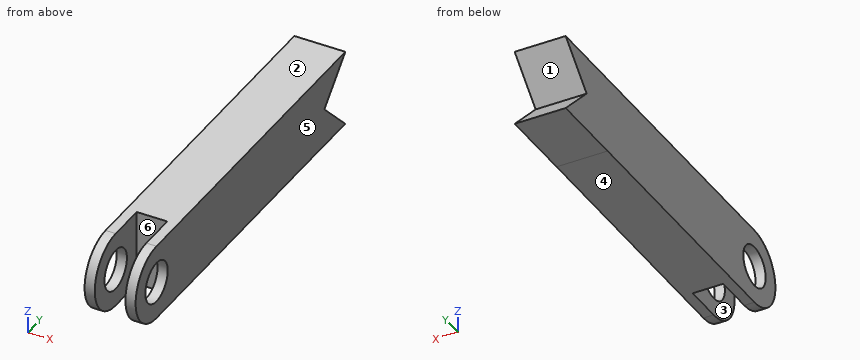
```python
from build123d import *

# Parameters (mm, degrees)
BOSS_EXTRUDE1_DEPTH = 100
CUT_EXTRUDE2_DEPTH  = 20
CUT_EXTRUDE3_START  = -20
CUT_EXTRUDE3_DEPTH  = 20
SKETCH10_R          = 40
BOSS_EXTRUDE6_DEPTH = 20
BOSS_EXTRUDE7_START = 20
SKETCH11_R          = 40
BOSS_EXTRUDE7_DEPTH = 20
SKETCH19_R          = 40
CUT_EXTRUDE7_DEPTH  = 285
SKETCH16_W          = 60
SKETCH16_H          = 150
CUT_EXTRUDE8_DEPTH  = 285
SKETCH20_W          = 100
SKETCH20_H          = 295.959975124
CUT_EXTRUDE9_DEPTH  = 285
BOSS_EXTRUDE8_DEPTH = 100


with BuildPart() as part:
    # Sketch1 → Boss-Extrude1 (new body)
    with BuildSketch(Plane(origin=(0, 0, 0), x_dir=(0, 0, -1), z_dir=(1, 0, 0))):
        with BuildLine():
            Line((-74.767803634, 0), (-74.767803634, 600))
            ThreePointArc((-74.767803634, 600), (0, 674.767803634), (74.767803634, 600))
            Line((74.767803634, 600), (74.767803634, 0))
            ThreePointArc((74.767803634, 0), (0, -74.767803634), (-74.767803634, 0))
        make_face()
    extrude(amount=BOSS_EXTRUDE1_DEPTH)

    # Sketch8 → Cut-Extrude2 (cut)
    with BuildSketch(Plane.ZY):
        with BuildLine():
            Line((-74.767803634, 600), (-74.767803634, 525))
            Line((-74.767803634, 525), (74.767803634, 525))
            Line((74.767803634, 525), (74.767803634, 600))
            ThreePointArc((74.767803634, 600), (0, 674.767803634), (-74.767803634, 600))
        make_face()
    extrude(amount=-CUT_EXTRUDE2_DEPTH, mode=Mode.SUBTRACT)

    # Sketch7 → Cut-Extrude3 (cut)
    with BuildSketch(Plane(origin=(100, 0, 0), x_dir=(0, 0, -1), z_dir=(1, 0, 0)).offset(CUT_EXTRUDE3_START)):
        with BuildLine():
            Line((-74.767803634, 600), (-74.767803634, 525))
            Line((-74.767803634, 525), (74.767803634, 525))
            Line((74.767803634, 525), (74.767803634, 600))
            ThreePointArc((74.767803634, 600), (0, 674.767803634), (-74.767803634, 600))
        make_face()
    extrude(amount=CUT_EXTRUDE3_DEPTH, mode=Mode.SUBTRACT)

    # Sketch10 → Boss-Extrude6 (add)
    with BuildSketch(Plane(origin=(80, 0, 0), x_dir=(0, 0, -1), z_dir=(1, 0, 0))):
        with Locations(Location((0, 600, 0), (0, 0, 180))):
            Circle(SKETCH10_R)
    extrude(amount=BOSS_EXTRUDE6_DEPTH)

    # Sketch11 → Boss-Extrude7 (add)
    with BuildSketch(Plane.ZY.offset(-20).offset(BOSS_EXTRUDE7_START)):
        with Locations((0, 600)):
            Circle(SKETCH11_R)
    extrude(amount=-BOSS_EXTRUDE7_DEPTH)

    # Sketch19 → Cut-Extrude7 (cut)
    with BuildSketch(Plane.ZY):
        Circle(SKETCH19_R)
    extrude(amount=-CUT_EXTRUDE7_DEPTH, mode=Mode.SUBTRACT)

    # Sketch16 → Cut-Extrude8 (cut)
    with BuildSketch(Plane.XY.offset(74.767803634)):
        with Locations((50, 0)):
            Rectangle(SKETCH16_W, SKETCH16_H)
    extrude(amount=-CUT_EXTRUDE8_DEPTH, mode=Mode.SUBTRACT)

    # Sketch20 → Cut-Extrude9 (cut)
    with BuildSketch(Plane.XY.offset(74.767803634)):
        with Locations((50, 672.979987562)):
            Rectangle(SKETCH20_W, SKETCH20_H)
    extrude(amount=-CUT_EXTRUDE9_DEPTH, mode=Mode.SUBTRACT)

    # Sketch21 → Boss-Extrude8 (add)
    with BuildSketch(Plane(origin=(100, 0, 0), x_dir=(0, 0, -1), z_dir=(1, 0, 0))):
        Polygon((-74.767803634, 525), (-74.767803634, 675), (0.232196366, 600), (75.232196366, 675), (74.767803634, 525), align=None)
    extrude(amount=-BOSS_EXTRUDE8_DEPTH)


solid = part.part
```
Source: CAD feature listing. Evaluate the final solid. Frame: model axes, mm. Face numbers are marked on the shaded views. A direction names the side the tool comes from. Give positions to 0.01 mm unless a question says otherwise; leave off trailing zeros. Loops run counter-clockwise (first coordinate to the right, second up) from the corner with the lowest first, then second, coordinate; pieces in that order, holes last. Notation, with made-up numbers: (-28.5, 14) -> (8.5, 14) arc R10 cw to (8.5, 22) -> close; hole circle Ø5 at (66, 49.5). An arc over 180 degrees is marked (long way). Put each result on its own line as item: value. Start each with the question number.
1) Cut plane C-C (z = -48). Return loops of the section in (x, y).
2) Cut plane B-B (z = -18.5). Return loops of the section in (x, y).
3) Material intervals for probe 1 along X at (y, z) = (-3, 41); probe 2 along Z at (x, y) = (73.5, 213); probe 3 along Y at (x, z) = (10, 0), sorted ascending.
4) Draft query along X for the marked faces 4, 5 and 6. Return one class per face: released by +X, released by -X, zero draft, split by the parting line, or undercut.
5) Cut plane D-D (x = 50). Return loops of the section in (y, z), then the cut area to 3 significant figures.
6) Contact query for flat-ended pins moving along their axis: P1, Ø12, axis at y = 508.5, z = 58.5, coming from the -X side; P2, Ø1.5, axis at x = 40, y = 190.5, coming from the -Z side; P3, Ø1, axis at x = 26.5, z = -22.5, coming from the +Y side. Output: stop coordinate, or through.
7) Reachability of the marked faces 1, 2 and 3 from +Z, -Z, +X, -X, +Y, -Y: full face, straight path, thin tool, end or side. Return the list, or none.
8) Cut plane A-A (x = 89). Return loops of the section in (y, z).
Results are:
1. outline: (0, -57.33) -> (20, -57.33) -> (20, 75) -> (80, 75) -> (80, -57.33) -> (100, -57.33) -> (100, 647.77) -> (0, 647.77) -> close
2. outline: (0, -72.44) -> (20, -72.44) -> (20, -35.46) -> (0, -35.46) -> close; (0, 35.46) -> (20, 35.46) -> (20, 75) -> (80, 75) -> (80, 35.46) -> (100, 35.46) -> (100, 618.27) -> (0, 618.27) -> close; (80, -72.44) -> (100, -72.44) -> (100, -35.46) -> (80, -35.46) -> close
3. probe 1: x = 0 to 20, 80 to 100
3. probe 2: z = -74.77 to 74.77
3. probe 3: y = -74.77 to -40, 40 to 600.23
4. face 4: zero draft
4. face 5: released by +X
4. face 6: undercut
5. outline: (75, -74.77) -> (525, -74.77) -> (675, -75.23) -> (600, -0.23) -> (675, 74.77) -> (75, 74.77) -> close
5. area: 84,100 mm2
6. P1: stops at x = 0
6. P2: stops at z = -74.77
6. P3: stops at y = 622.77
7. face 1: +X, -X, +Y
7. face 2: +Z, +X, -X, +Y, -Y
7. face 3: +Z, -Z, -Y
8. outline: (0, -74.77) -> (525, -74.77) -> (675, -75.23) -> (600, -0.23) -> (675, 74.77) -> (0, 74.77) arc R74.77 ccw to start; hole circle Ø80 at (0, 0)
